For this review, take the finished solid that the model builds, in its own axes (mm). Face numbers are marked on the shaded views. A direction names the side the tool comes from. Coordinates: 2 decimals unless noted, no trailing zeros. Loops run counter-clockwise (first coordinate to the right, second up) from the corner with the lowest first, then second, coordinate; pieces in that order, holes last. Notation, with made-up numbers: (80.5, 54) -> (107.5, 54) arc R10 ccw to (107.5, 67) -> close; hole circle Ø9 at (-32.5, 9). An arc over 180 degrees is marked (long way). One line per item, written item: value.
Autodesk Inventor part; units mm, degrees
ref_plane "YZ Plane" through (0, 0, 0) normal (1, 0, 0) x (0, 1, 0)
ref_plane "XZ Plane" through (0, 0, 0) normal (0, 1, 0) x (-1, 0, 0)
ref_plane "XY Plane" through (0, 0, 0) normal (0, 0, 1) x (1, 0, 0)
sketch "Sketch1" plane through (0, 0, 0) normal (0, 0, 1) x (1, 0, 0)
  line L0 (0, 0) -> (25.4, 0)
  line L1 (25.4, 0) -> (25.4, 19.05)
  line L2 (25.4, 19.05) -> (0, 19.05)
  line L3 (0, 19.05) -> (0, 0)
  dimension "d0" = 25.4
  dimension "d1" = 19.05
extrude "Extrusion1" add sketch "Sketch1" along normal blind 76.2
sketch "Sketch2" plane through (25.4, 0, 0) normal (1, 0, 0) x (0, 0, -1)
  line L0 (0, 0) -> (0, 19.05)
  line L1 (0, 19.05) -> (-76.2, 19.05)
  point P0 (-51.6636, 9.525)
  point P1 (-24.5364, 9.525)
  dimension "d4" = 27.1272
  dimension "d6" = 9.525
  dimension "d7" = 9.525
  dimension "d29" = 24.5364
hole "Hole1" at (25.4, 9.525, 51.6636) at (25.4, 9.525, 24.5364) direction (-1, 0, 0) diameter 4.9784 depth 22.225 tip angle 118
sketch "Sketch3" plane through (0, 19.05, 0) normal (0, 1, 0) x (1, 0, 0)
  line L0 (6.35, -12.7) -> (19.05, -12.7) construction
  line L1 (6.35, -16.002) -> (19.05, -16.002)
  line L2 (19.05, -9.398) -> (6.35, -9.398)
  arc A0 (6.35, -9.398) -> (6.35, -16.002) centre (6.35, -12.7) ccw
  arc A1 (19.05, -16.002) -> (19.05, -9.398) centre (19.05, -12.7) ccw
  line L3 (6.35, -63.5) -> (19.05, -63.5) construction
  line L4 (6.35, -66.802) -> (19.05, -66.802)
  line L5 (19.05, -60.198) -> (6.35, -60.198)
  arc A2 (6.35, -60.198) -> (6.35, -66.802) centre (6.35, -63.5) ccw
  arc A3 (19.05, -66.802) -> (19.05, -60.198) centre (19.05, -63.5) ccw
  line L6 (6.35, -38.1) -> (19.05, -38.1) construction
  line L7 (6.35, -41.402) -> (19.05, -41.402)
  line L8 (19.05, -34.798) -> (6.35, -34.798)
  arc A4 (6.35, -34.798) -> (6.35, -41.402) centre (6.35, -38.1) ccw
  arc A5 (19.05, -41.402) -> (19.05, -34.798) centre (19.05, -38.1) ccw
  line L9 (25.4, 0) -> (25.4, -76.2)
  line L10 (25.4, -76.2) -> (0, -76.2)
  point P0 (12.7, -12.7)
  point P1 (12.7, -63.5)
  point P2 (12.7, -38.1)
  dimension "d15" = 3.302
  dimension "d16" = 3.302
  dimension "d17" = 3.302
  dimension "d18" = 12.7
  dimension "d19" = 12.7
  dimension "d20" = 12.7
  dimension "d21" = 25.4
  dimension "d22" = 25.4
  dimension "d23" = 6.35
  dimension "d24" = 6.35
  dimension "d25" = 6.35
  dimension "d26" = 12.7
extrude "Extrusion2" cut sketch "Sketch3" against normal blind 101.6
properties part number "Motor Base" material "Aluminum 6061"
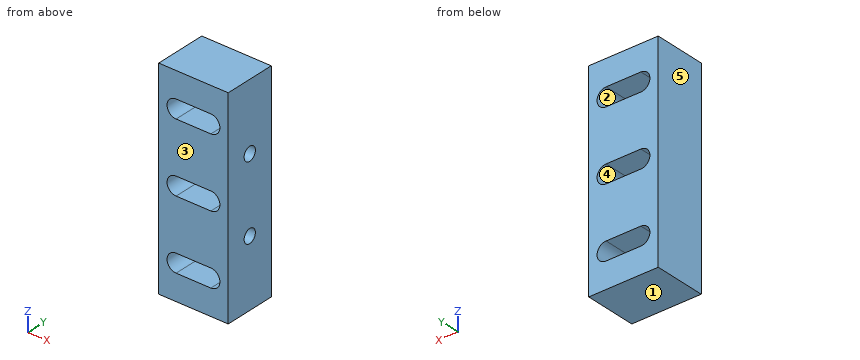
1. Take a section at B-B, the plane y = 4.75. Give the boundary of the cut face in (x, z).
Return value:
outline: (0, 0) -> (25.4, 0) -> (25.4, 76.2) -> (0, 76.2) -> close; hole (6.35, 9.4) -> (19.05, 9.4) arc R3.3 ccw to (19.05, 16) -> (6.35, 16) arc R3.3 ccw to start; hole (6.35, 34.8) -> (19.05, 34.8) arc R3.3 ccw to (19.05, 41.4) -> (6.35, 41.4) arc R3.3 ccw to start; hole (6.35, 60.2) -> (19.05, 60.2) arc R3.3 ccw to (19.05, 66.8) -> (6.35, 66.8) arc R3.3 ccw to start
2. For the marked faces 4 and 5, list the 3-axis set-ups (+Z, -Z, +X, -X, +Y, -Y) from which the entire face can be reached by the end or side of a thin tool; tool diameter is ignored.
Return value:
face 4: +Y, -Y
face 5: +Z, -Z, -X, +Y, -Y
3. Take a section at C-C, the plane x = 4.5. Give the boundary of the cut face in (y, z) (3 decimals), and give its area (3 significant figures).
Return value:
outline: (0, 0) -> (19.05, 0) -> (19.05, 9.965) -> (0, 9.965) -> close; (0, 15.435) -> (19.05, 15.435) -> (19.05, 35.365) -> (0, 35.365) -> close; (0, 40.835) -> (19.05, 40.835) -> (19.05, 60.765) -> (0, 60.765) -> close; (0, 66.235) -> (19.05, 66.235) -> (19.05, 76.2) -> (0, 76.2) -> close; hole circle Ø4.978 at (9.525, 24.536); hole circle Ø4.978 at (9.525, 51.664)
area: 1,100 mm2
4. Take a section at A-A, the plane z = 12.7. Give the boundary of the cut face in (x, y).
Return value:
outline: (0, 0) -> (3.05, 0) -> (3.05, 19.05) -> (0, 19.05) -> close; (22.35, 0) -> (25.4, 0) -> (25.4, 19.05) -> (22.35, 19.05) -> close
5. To check wall thickness, follow probe 1 along Z at (x, y) = (17.5, 17.5); probe 2 along Z at (x, y) = (15.5, 9.5); probe 3 along Z at (x, y) = (4, 13.75). State the ranges of each line that lie inside material, in increasing order. Write a range as from..to.
Return value:
probe 1: z = 0..9.4, 16..34.8, 41.4..60.2, 66.8..76.2
probe 2: z = 0..9.4, 16..22.05, 27.03..34.8, 41.4..49.17, 54.15..60.2, 66.8..76.2
probe 3: z = 0..10.38, 15.02..35.78, 40.42..61.18, 65.82..76.2
6. The part is to be moulded in two halves that separate along Z. For the marked faces 1, 2 and 3, say which applies: pulls with the +Z half, pulls with the -Z half, needs draft (parallel to the pull), parting line crosses it, or undercut.
Return value:
face 1: pulls with the -Z half
face 2: undercut
face 3: needs draft
7. Take a section at D-D, the plane x = 23.25. Give the boundary of the cut face in (y, z) (3 decimals), and give its area (3 significant figures).
Return value:
outline: (0, 0) -> (19.05, 0) -> (19.05, 76.2) -> (0, 76.2) -> close; hole circle Ø4.978 at (9.525, 24.536); hole circle Ø4.978 at (9.525, 51.664)
area: 1,410 mm2
